from build123d import *

# Parameters (mm, degrees)
SKETCH1_W      = 50.8
SKETCH1_H      = 265.43
SKETCH1_R      = 3.175
EXTRUDE1_DEPTH = 3.175
FILLET1_R      = 3.175


with BuildPart() as part:
    # Sketch1 → Extrude1 (new, symmetric)
    with BuildSketch(Plane.XY):
        Rectangle(SKETCH1_W, SKETCH1_H)
        with Locations((0, 106.35742)):
            Circle(SKETCH1_R, mode=Mode.SUBTRACT)
        with Locations((0, 96.19742)):
            Circle(SKETCH1_R, mode=Mode.SUBTRACT)
        with Locations((0, 15.24)):
            Circle(SKETCH1_R, mode=Mode.SUBTRACT)
        with Locations((0, 25.4)):
            Circle(SKETCH1_R, mode=Mode.SUBTRACT)
        with Locations((12.7, -120.015)):
            Circle(SKETCH1_R, mode=Mode.SUBTRACT)
        with Locations((-12.7, -120.015)):
            Circle(SKETCH1_R, mode=Mode.SUBTRACT)
        with BuildLine():
            Line((9.525, 73.49871), (9.525, 48.09871))
            ThreePointArc((9.525, 48.09871), (0, 38.57371), (-9.525, 48.09871))
            Line((-9.525, 48.09871), (-9.525, 73.49871))
            ThreePointArc((-9.525, 73.49871), (0, 83.02371), (9.525, 73.49871))
        make_face(mode=Mode.SUBTRACT)
    extrude(amount=EXTRUDE1_DEPTH, both=True)

    # Fillet1
    fillet1_edges = [part.edges().sort_by_distance(p)[0] for p in [
        (-25.4, 132.715, 0),
        (25.4, 132.715, 0),
    ]]
    fillet(fillet1_edges, radius=FILLET1_R)


solid = part.part
Here's how the part is built. I have some questions about the finished solid (model axes, mm). A direction names the side the tool comes from. Round coordinates to 2 decimals unless told otherwise and drop trailing zeros. Order: outer loops, then holes, each group sorted by start corner. A loop starts at its lowest first (then second) coordinate and runs counter-clockwise, first axis right, second up. Notation, with made-up numbers: M -25.75,43.25 L -11.75,43.25 A18 ccw -11.75,72.25 Z; hole C -28.75,-4.75 d5. An arc over 180 degrees is marked long. Return JSON: item names as keys, results as strings. Group by question number.
1. On a 3-axis mill with a long thin cutter (end or side, diameter ignored), from which of +Z, -Z, +X, -X, +Y, -Y can I reach the whole of each face in a straight line? I mean faces 1 (the face through (9.525, 61, 0)), 2 (the face through (0, 132.715, 0)). Say none if no direction works.
2. Please list where these lines run through material, in increasing order: probe 1 along Y at (x, z) = (0, -1.5) (3 decimals); probe 2 along Y at (x, z) = (12.7, 1) (3 decimals); probe 3 along X at (y, z) = (15.5, 0.5).
3. If we section it at A-A on x = 0: List the corners of the cut face in (y, z) for me (3 decimals), then the cut area to 3 significant figures.
4. If we mould it in two halves opening along X, with no side actions, what happens to faces 3 (the face through (12.012, -123.114, -0.044)), 4 (the face through (25.4, -3, 0)), 5 (the face through (0, 2, 3.175))? For each: pulls with the +X half, pulls with the -X half, needs draft (parallel to the pull), parting line crosses it, or undercut.
5. If we section it at D-D on z = 1: List the corners of the cut face in (x, y) for me (3 decimals), then the cut area to 3 significant figures.
6. I'm going to push a flat-ended pin straight in: pin 1 Ø5.5 at (x, y) = (0, 15.24) entering from -Z. Where does the tip first touch, or does it pass through?
7. If we section it at B-B on y = 25.4: List the corners of the cut face in (x, z) for me (3 decimals).
8. If we section it at C-C on x = -12.7: List the corners of the cut face in (y, z) for me (3 decimals).
Reply:
{
 "1": {"face 1": "+Z, -Z", "face 2": "+Z, -Z, +X, -X, +Y"},
 "2": {"probe 1": "-132.715 to 12.065, 18.415 to 22.225, 28.575 to 38.574, 83.024 to 93.022, 99.372 to 103.182, 109.532 to 132.715", "probe 2": "-132.715 to -123.19, -116.84 to 132.715", "probe 3": "-25.4 to -3.16, 3.16 to 25.4"},
 "3": {"outline": "M -132.715,-3.175 L 12.065,-3.175 L 12.065,3.175 L -132.715,3.175 Z; M 18.415,-3.175 L 22.225,-3.175 L 22.225,3.175 L 18.415,3.175 Z; M 28.575,-3.175 L 38.574,-3.175 L 38.574,3.175 L 28.575,3.175 Z; M 83.024,-3.175 L 93.022,-3.175 L 93.022,3.175 L 83.024,3.175 Z; M 99.372,-3.175 L 103.182,-3.175 L 103.182,3.175 L 99.372,3.175 Z; M 109.532,-3.175 L 132.715,-3.175 L 132.715,3.175 L 109.532,3.175 Z", "area": "1,240 mm^2"},
 "4": {"face 3": "undercut", "face 4": "pulls with the +X half", "face 5": "needs draft"},
 "5": {"outline": "M -25.4,-132.715 L 25.4,-132.715 L 25.4,129.54 A3.175 ccw 22.225,132.715 L -22.225,132.715 A3.175 ccw -25.4,129.54 Z; hole C -12.7,-120.015 d6.35; hole M -9.525,48.099 A9.525 ccw 9.525,48.099 L 9.525,73.499 A9.525 ccw -9.525,73.499 Z; hole C 0,15.24 d6.35; hole C 0,25.4 d6.35; hole C 0,96.197 d6.35; hole C 0,106.357 d6.35; hole C 12.7,-120.015 d6.35", "area": "12,500 mm^2"},
 "6": {"pin 1": "through"},
 "7": {"outline": "M -25.4,-3.175 L -3.175,-3.175 L -3.175,3.175 L -25.4,3.175 Z; M 3.175,-3.175 L 25.4,-3.175 L 25.4,3.175 L 3.175,3.175 Z"},
 "8": {"outline": "M -132.715,-3.175 L -123.19,-3.175 L -123.19,3.175 L -132.715,3.175 Z; M -116.84,-3.175 L 132.715,-3.175 L 132.715,3.175 L -116.84,3.175 Z"}
}
